Check sheet for the modelled part. Datum: model origin and axes. Units: mm. A direction names the side the tool comes from. Give positions to 0.01 mm unless a question says otherwise; leave off trailing zeros. Loops run counter-clockwise (first coordinate to the right, second up) from the corner with the lowest first, then second, coordinate; pieces in that order, holes last. Notation, with made-up numbers: (-40, 65.25) - (14, 65.25) arc R13 ccw to (14, 89.25) - close; hole circle Ø8 at (-5.5, 14.25). An arc over 180 degrees is marked (long way). Answer in a Markdown table with one row per item. Add a question column.
(1) Sectioned sample at A-A on x = 18.5. Enter the section's corners in (y, z), then the cut area to 3 significant figures.
(2) Draft check along X on faces 1 (the face through (8.462, -0.172, 8.913)), 2 (the face through (-7.139, 13.158, 15.662)), 3 (the face through (19, -7, 4)), 4 (the face through (22.88, -2.24, 3.29)). Enter one of: released by +X, released by -X, zero draft, split by the parting line, or undercut.
(3) Thickness scan on L1, parallel to X at y = 0.5, z = 12.5; L2, parallel to Z at x = -16.5, y = 12.5; L3, parallel to Y at x = 2, z = 17.5. Record the ranges inside material, lowest first.
(4) Sectioned sample at B-B on y = -10.25. Enter the section's corners in (x, z).
(5) Go/stop test with flat-tipped pins: P1, Ø7.5, axis at y = 0, z = 4, coming from the -X side; P2, Ø2.5, axis at y = 0.5, z = 4, coming from the +X side; P3, Ø1.4, axis at x = -18.5, z = 5, coming from the -Y side; P4, Ø2.5, axis at y = 0, z = 4, coming from the +X side. Record where each tip stops, or that it passes through.
(6) Sectioned sample at D-D on x = 0. Enter the section's corners in (y, z), then the cut area to 3 significant figures.
(7) Sectioned sample at C-C on z = 16. Enter the section's corners in (x, y).
(8) Set-up check for faces 5 (the face through (1.21, 12.147, 18.422)), 6 (the face through (-17, -11, 4)), 7 (the face through (0, 13.5, 16)), 8 (the face through (19, 8.8, 4)): record each of +Z, -Z, +X, -X, +Y, -Y from which the full face is reachable in a straight line by a thin tool's end or side.
from build123d import *

# Parameters (mm, degrees)
ESQUISSE1_W                = 49
ESQUISSE1_H                = 34
BASE_DEPTH                 = 8
ESQUISSE2_R                = 2.35
INSERT_M3_L_DEPTH          = 3.2
INSERT_M3_R_START          = -3.2
ESQUISSE3_R                = 2.35
INSERT_M3_R_DEPTH          = 3.2
ESQUISSE4_R                = 2.35
INSERT_M3_TOP_DEPTH        = 3.2
INSER_M3_BOT_START         = 3.2
ESQUISSE5_R                = 2.35
INSER_M3_BOT_DEPTH         = 3.2
ESQUISSE11_R               = 1.5
PASSAGE_VIS_L_DEPTH        = 5
PASSAGE_VIS_R_START        = -5
ESQUISSE12_R               = 1.5
PASSAGE_VIS_R_DEPTH        = 5
ESQUISSE10_R               = 1.5
PASSAGE_VIS_TOP_DEPTH      = 5
PASSAGE_VIS_BOT_START      = -5
ESQUISSE13_R               = 1.5
PASSAGE_VIS_BOT_DEPTH      = 5
CONG_1_R                   = 1.2
ESQUISSE6_W                = 15
ESQUISSE6_H                = 27
SUPPORT_FIXATION_DEPTH     = 12
PASSAGE_GUIDON_REACH       = 43.388
CONG_VERTICAL_R            = 1.2
CONG_BASE_R                = 3.2
ESQUISSE8_R                = 2.25
INSERTS_M3_FIXATION_DEPTH  = 3.2
ESQUISSE9_R                = 1.5
PASSAGE_VIS_FIXATION_DEPTH = 5
PASSE_CABLE_DEPTH          = 8


with BuildPart() as part:
    # Esquisse1 → Base (new body)
    with BuildSketch(Plane.XY):
        Rectangle(ESQUISSE1_W, ESQUISSE1_H)
    extrude(amount=BASE_DEPTH)

    # Esquisse2 → Insert_M3_L (cut)
    with BuildSketch(Plane.ZY.offset(24.5)):
        with Locations(Location((4, 0, 0), (0, 0, 270))):
            Circle(ESQUISSE2_R)
    extrude(amount=-INSERT_M3_L_DEPTH, mode=Mode.SUBTRACT)

    # Esquisse3 → Insert_M3_R (cut)
    with BuildSketch(Plane(origin=(24.5, 0, 0), x_dir=(0, 0, -1), z_dir=(1, 0, 0)).offset(INSERT_M3_R_START)):
        with Locations(Location((-4, 0, 0), (0, 0, 270))):
            Circle(ESQUISSE3_R)
    extrude(amount=INSERT_M3_R_DEPTH, mode=Mode.SUBTRACT)

    # Esquisse4 → Insert_M3_TOP (cut)
    with BuildSketch(Plane(origin=(0, 17, 0), x_dir=(1, 0, 0), z_dir=(0, 1, 0))):
        with Locations(Location((-18.5, -4, 0), (0, 0, 180))):
            Circle(ESQUISSE4_R)
        with Locations(Location((18.5, -4, 0), (0, 0, 180))):
            Circle(ESQUISSE4_R)
    extrude(amount=-INSERT_M3_TOP_DEPTH, mode=Mode.SUBTRACT)

    # Esquisse5 → Inser_M3_BOT (cut)
    with BuildSketch(Plane(origin=(0, -17, -17), x_dir=(1, 0, 0), z_dir=(0, 1, 0)).offset(INSER_M3_BOT_START)):
        with Locations(Location((-18.5, -21, 0), (0, 0, 180))):
            Circle(ESQUISSE5_R)
        with Locations(Location((18.5, -21, 0), (0, 0, 180))):
            Circle(ESQUISSE5_R)
    extrude(amount=-INSER_M3_BOT_DEPTH, mode=Mode.SUBTRACT)

    # Esquisse11 → Passage_Vis_L (cut)
    with BuildSketch(Plane.ZY.offset(21.3)):
        with Locations(Location((4, 0, 0), (0, 0, 270))):
            Circle(ESQUISSE11_R)
    extrude(amount=-PASSAGE_VIS_L_DEPTH, mode=Mode.SUBTRACT)

    # Esquisse12 → Passage_Vis_R (cut)
    with BuildSketch(Plane(origin=(21.3, 0, 0), x_dir=(0, 0, -1), z_dir=(1, 0, 0)).offset(PASSAGE_VIS_R_START)):
        with Locations(Location((-4, 0, 0), (0, 0, 270))):
            Circle(ESQUISSE12_R)
    extrude(amount=PASSAGE_VIS_R_DEPTH, mode=Mode.SUBTRACT)

    # Esquisse10 → Passage_Vis_TOP (cut)
    with BuildSketch(Plane(origin=(0, 13.8, 0), x_dir=(1, 0, 0), z_dir=(0, 1, 0))):
        with Locations(Location((-18.5, -4, 0), (0, 0, 180))):
            Circle(ESQUISSE10_R)
        with Locations(Location((18.5, -4, 0), (0, 0, 180))):
            Circle(ESQUISSE10_R)
    extrude(amount=-PASSAGE_VIS_TOP_DEPTH, mode=Mode.SUBTRACT)

    # Esquisse13 → Passage_Vis_BOT (cut)
    with BuildSketch(Plane.XZ.offset(13.8).offset(PASSAGE_VIS_BOT_START)):
        with Locations(Location((-18.5, 4, 0), (0, 0, 180))):
            Circle(ESQUISSE13_R)
        with Locations(Location((18.5, 4, 0), (0, 0, 180))):
            Circle(ESQUISSE13_R)
    extrude(amount=PASSAGE_VIS_BOT_DEPTH, mode=Mode.SUBTRACT)

    # Congé1
    cong_1_edges = [part.edges().sort_by_distance(p)[0] for p in [
        (-24.5, 17, 4),
        (24.5, 17, 4),
        (24.5, -17, 4),
        (-24.5, -17, 4),
    ]]
    fillet(cong_1_edges, radius=CONG_1_R)

    # Esquisse6 → Support_Fixation (add)
    with BuildSketch(Plane.XY.offset(8)):
        Rectangle(ESQUISSE6_W, ESQUISSE6_H)
    extrude(amount=SUPPORT_FIXATION_DEPTH)

    # Esquisse7 → Passage_Guidon (cut, up to next)
    with BuildSketch(Plane.ZY.offset(7.5), mode=Mode.PRIVATE) as passage_guidon_sk1:
        with BuildLine():
            Line((20, 7), (20, -7))
            ThreePointArc((20, -7), (13, 0), (20, 7))
        make_face()
    passage_guidon_tool1 = extrude(passage_guidon_sk1.sketch, amount=-PASSAGE_GUIDON_REACH, mode=Mode.PRIVATE) & part.part
    add(passage_guidon_tool1.solids().sort_by_distance((-7.5, 0, 17.029108))[0], mode=Mode.SUBTRACT)

    # Congé_Vertical
    cong_vertical_edges = [part.edges().sort_by_distance(p)[0] for p in [
        (-7.5, 13.5, 14),
        (-7.5, -13.5, 14),
        (7.5, -13.5, 14),
        (7.5, 13.5, 14),
    ]]
    fillet(cong_vertical_edges, radius=CONG_VERTICAL_R)

    # Congé_Base
    cong_base_edges = [part.edges().sort_by_distance(p)[0] for p in [
        (-7.5, 0, 8),
        (0, 13.5, 8),
        (7.5, 0, 8),
        (0, -13.5, 8),
        (-7.148528137, 13.148528137, 8),
        (7.148528137, 13.148528137, 8),
        (7.148528137, -13.148528137, 8),
        (-7.148528137, -13.148528137, 8),
    ]]
    fillet(cong_base_edges, radius=CONG_BASE_R)

    # Esquisse8 → Inserts_M3_Fixation (cut)
    with BuildSketch(Plane.XY.offset(20)):
        with Locations((0, 10.25)):
            Circle(ESQUISSE8_R)
        with Locations(Location((0, -10.25, 0), (0, 0, 180))):
            Circle(ESQUISSE8_R)
    extrude(amount=-INSERTS_M3_FIXATION_DEPTH, mode=Mode.SUBTRACT)

    # Esquisse9 → Passage_Vis_Fixation (cut)
    with BuildSketch(Plane.XY.offset(16.8)):
        with Locations((0, 10.25)):
            Circle(ESQUISSE9_R)
        with Locations(Location((0, -10.25, 0), (0, 0, 180))):
            Circle(ESQUISSE9_R)
    extrude(amount=-PASSAGE_VIS_FIXATION_DEPTH, mode=Mode.SUBTRACT)

    # Esquisse14 → Passe_Cable (cut)
    with BuildSketch(Plane.XY.offset(8)):
        with BuildLine():
            Line((16.5, -3.9), (20.7, -3.9))
            ThreePointArc((20.7, -3.9), (21.407106781, -4.192893219), (21.7, -4.9))
            Line((21.7, -4.9), (21.7, -6))
            ThreePointArc((21.7, -6), (21.407106781, -6.707106781), (20.7, -7))
            Line((20.7, -7), (16.5, -7))
            ThreePointArc((16.5, -7), (15.792893219, -6.707106781), (15.5, -6))
            Line((15.5, -6), (15.5, -4.9))
            ThreePointArc((15.5, -4.9), (15.792893219, -4.192893219), (16.5, -3.9))
        make_face()
    extrude(amount=-PASSE_CABLE_DEPTH, mode=Mode.SUBTRACT)


solid = part.part
Reply:
| question | item | result |
|---|---|---|
| 1 | outline | (-17, 0) - (-7, 0) - (-7, 8) - (-17, 8) - (-17, 6.35) - (-13.8, 6.35) - (-13.8, 5.5) - (-8.8, 5.5) - (-8.8, 2.5) - (-13.8, 2.5) - (-13.8, 1.65) - (-17, 1.65) - close; (-3.9, 0) - (17, 0) - (17, 1.65) - (13.8, 1.65) - (13.8, 2.5) - (8.8, 2.5) - (8.8, 5.5) - (13.8, 5.5) - (13.8, 6.35) - (17, 6.35) - (17, 8) - (-3.9, 8) - close; hole circle Ø3 at (0, 4) |
| 1 | area | 180 mm^2 |
| 2 | face 1 | released by +X |
| 2 | face 2 | released by -X |
| 2 | face 3 | undercut |
| 2 | face 4 | zero draft |
| 3 | L1 | -7.5 to 7.5 |
| 3 | L2 | 0 to 8 |
| 3 | L3 | -13.5 to -11.28, -9.22 to -6.54, 6.54 to 9.22, 11.28 to 13.5 |
| 4 | outline | (-24.5, 0) - (24.5, 0) - (24.5, 8) - (10.7, 8) arc R3.2 cw to (7.5, 11.2) - (7.5, 20) - (2.25, 20) - (2.25, 16.8) - (1.5, 16.8) - (1.5, 11.8) - (-1.5, 11.8) - (-1.5, 16.8) - (-2.25, 16.8) - (-2.25, 20) - (-7.5, 20) - (-7.5, 11.2) arc R3.2 cw to (-10.7, 8) - (-24.5, 8) - close; hole circle Ø3 at (-18.5, 4); hole circle Ø3 at (18.5, 4) |
| 5 | P1 | x = -24.5 |
| 5 | P2 | x = 21.3 |
| 5 | P3 | y = -13.8 |
| 5 | P4 | x = 16.3 |
| 6 | outline | (-17, 0) - (17, 0) - (17, 8) - (16.7, 8) arc R3.2 cw to (13.5, 11.2) - (13.5, 20) - (12.5, 20) - (12.5, 16.8) - (11.75, 16.8) - (11.75, 11.8) - (8.75, 11.8) - (8.75, 16.8) - (8, 16.8) - (8, 20) - (7, 20) arc R7 cw to (-7, 20) - (-8, 20) - (-8, 16.8) - (-8.75, 16.8) - (-8.75, 11.8) - (-11.75, 11.8) - (-11.75, 16.8) - (-12.5, 16.8) - (-12.5, 20) - (-13.5, 20) - (-13.5, 11.2) arc R3.2 cw to (-16.7, 8) - (-17, 8) - close |
| 6 | area | 465 mm^2 |
| 7 | outline | (-7.5, -12.3) arc R1.2 ccw to (-6.3, -13.5) - (6.3, -13.5) arc R1.2 ccw to (7.5, -12.3) - (7.5, -5.74) - (-7.5, -5.74) - close; (-7.5, 5.74) - (7.5, 5.74) - (7.5, 12.3) arc R1.2 ccw to (6.3, 13.5) - (-6.3, 13.5) arc R1.2 ccw to (-7.5, 12.3) - close; hole circle Ø3 at (0, -10.25); hole circle Ø3 at (0, 10.25) |
| 8 | face 5 | +Z |
| 8 | face 6 | -Y |
| 8 | face 7 | +Z, +X, -X, +Y |
| 8 | face 8 | +Y |
